from build123d import *

# Parameters (mm, degrees)
SKETCH1_W           = 214
SKETCH1_H           = 214
SKETCH1_R           = 1.6
BOSS_EXTRUDE1_DEPTH = 1.5
SKETCH2_W           = 86
SKETCH2_H           = 12
CUT_EXTRUDE1_DEPTH  = 2.5
FILLET1_R           = 4


with BuildPart() as part:
    # Sketch1 → Boss-Extrude1 (new body)
    with BuildSketch(Plane.XY):
        Rectangle(SKETCH1_W, SKETCH1_H)
        with Locations((-104.5, 104.5)):
            Circle(SKETCH1_R, mode=Mode.SUBTRACT)
        with Locations((104.5, 104.5)):
            Circle(SKETCH1_R, mode=Mode.SUBTRACT)
        with Locations((0, -104.5)):
            Circle(SKETCH1_R, mode=Mode.SUBTRACT)
        with Locations((104.5, -104.5)):
            Circle(SKETCH1_R, mode=Mode.SUBTRACT)
        with Locations((-104.5, -104.5)):
            Circle(SKETCH1_R, mode=Mode.SUBTRACT)
    extrude(amount=BOSS_EXTRUDE1_DEPTH)

    # Sketch2 → Cut-Extrude1 (cut, through all)
    with BuildSketch(Plane.XY.offset(1.5)):
        with Locations((0, -101)):
            Rectangle(SKETCH2_W, SKETCH2_H)
    extrude(amount=-CUT_EXTRUDE1_DEPTH, mode=Mode.SUBTRACT)

    # Fillet1
    fillet1_edges = [part.edges().sort_by_distance(p)[0] for p in [
        (-43, -95, 0.75),
        (43, -95, 0.75),
    ]]
    fillet(fillet1_edges, radius=FILLET1_R)


solid = part.part
The listing builds one solid part. Answer for the finished solid, in the listing's coordinates (mm). Coordinates: 2 decimals unless noted, no trailing zeros. Loops run counter-clockwise (first coordinate to the right, second up) from the corner with the lowest first, then second, coordinate; pieces in that order, holes last.
1) Find the intervals of material crossed by L1, parallel to Y at x = -104.5, z = 1.15; L2, parallel to X at y = -104.5, z = 0.55, in increasing order.
2) Find section B-B on x = -22.5. Write down the section's boundary in (y, z).
3) Find section A-A on z = 1.05. Write down the section's boundary in (x, y).
4) A flat-ended cylindrical pin translates along its axis: pin 1 Ø0.8 at (x, z) = (-16.5, 1) entering from -Y. Find the tip coordinate at first contact, or state that the pin passes through.
Values:
1. L1: y = -107 to -106.1, -102.9 to 102.9, 106.1 to 107
1. L2: x = -107 to -106.1, -102.9 to -43, 43 to 102.9, 106.1 to 107
2. outline: (-95, 0) - (107, 0) - (107, 1.5) - (-95, 1.5) - close
3. outline: (-107, -107) - (-43, -107) - (-43, -99) arc R4 cw to (-39, -95) - (39, -95) arc R4 cw to (43, -99) - (43, -107) - (107, -107) - (107, 107) - (-107, 107) - close; hole circle Ø3.2 at (-104.5, -104.5); hole circle Ø3.2 at (-104.5, 104.5); hole circle Ø3.2 at (104.5, -104.5); hole circle Ø3.2 at (104.5, 104.5)
4. pin 1: stops at y = -95
